Source: CAD feature listing. Evaluate the final solid. Frame: model axes, mm. A direction names the side the tool comes from. Coordinates: 2 decimals unless noted, no trailing zeros. Order: outer loops, then holes, each group sorted by start corner. A loop starts at its lowest first (then second) coordinate and runs counter-clockwise, first axis right, second up.
```python
from build123d import *

# Parameters (mm, degrees)
SKETCH1_W          = 9.5
SKETCH1_H          = 2
SKETCH1_W_2        = 9
SKETCH1_H_2        = 7
SKETCH2_W          = 4
SKETCH2_H          = 0.5
CUT_EXTRUDE1_DEPTH = 8
SKETCH3_R          = 1.25
CUT_EXTRUDE2_DEPTH = 8


with BuildPart() as part:
    # Sketch1 → Revolve1 (revolve)
    with BuildSketch(Plane.XY, mode=Mode.PRIVATE) as revolve1_sk:
        with Locations((-4.75, 1)):
            Rectangle(SKETCH1_W, SKETCH1_H)
        Polygon((0, 2), (0, 0), (21.5, 0), (21.5, 12.2), (21.5, 12.5), (2.5, 12.5), (2.5, 3.5), (0, 3.5), align=None)
        Polygon((21.5, 12.2), (21.5, 0), (52.5, 0), (52.5, 7), (52.5, 12.2), align=None)
        with Locations((57, 3.5)):
            Rectangle(SKETCH1_W_2, SKETCH1_H_2)
    revolve(revolve1_sk.sketch.rotate(Axis((0, 0, 0), (1, 0, 0)), 90), axis=Axis((0, 0, 0), (1, 0, 0)))

    # Sketch2 → Cut-Extrude1 (cut)
    with BuildSketch(Plane.ZY.offset(9.5)):
        with Locations((0, 1.75)):
            Rectangle(SKETCH2_W, SKETCH2_H)
    extrude(amount=-CUT_EXTRUDE1_DEPTH, mode=Mode.SUBTRACT)

    # Sketch3 → Cut-Extrude2 (cut)
    with BuildSketch(Plane.ZY.offset(-2.5)):
        with Locations((0, 8.5)):
            Circle(SKETCH3_R)
        with Locations(Location((0, -8.5, 0), (0, 0, 180))):
            Circle(SKETCH3_R)
    extrude(amount=-CUT_EXTRUDE2_DEPTH, mode=Mode.SUBTRACT)


solid = part.part
```
1. Section query D-D on z = -10. Return loops of the section in (x, y).
Findings:
outline: (2.5, -7.5) - (21.5, -7.5) - (21.5, -6.99) - (52.5, -6.99) - (52.5, 6.99) - (21.5, 6.99) - (21.5, 7.5) - (2.5, 7.5) - close
2. Access query for faces 1 (the face through (-9.5, 0, 0)), 2 (the face through (57.06, 6.21, 3.23)), 3 (the face through (10.5, 9, 0)). Directions: +Z, -Z, +X, -X, +Y, -Y. A direction counts if a zero-diameter tool reaches every point of the face in a straight line with its end or side. Return the directions, or none.
Findings:
face 1: +Z, -Z, -X, +Y, -Y
face 2: +X
face 3: -X
3. Draft query along Z for faces 4 (the face through (6.444, 9.554, 0.672)), 5 (the face through (-6, 1.5, 0)), 6 (the face through (36.8, 7.4, -9.7)). Return one class per face: released by +Z, released by -Z, zero draft, split by the parting line, or undercut.
Findings:
face 4: undercut
face 5: zero draft
face 6: split by the parting line
4. Section query C-C on x = 14. Return loops of the section in (y, z).
Findings:
outline: circle Ø25 at (0, 0)
5. Ray query, line 1 (Y direction, x = 6, z = 0); line 2 (X direction, y = 9, z = 2.5); line 3 (X direction, y = -3, z = -0.5). Return the intervals inside material, ascending.
Findings:
line 1: y = -12.5 to -9.75, -7.25 to 7.25, 9.75 to 12.5
line 2: x = 2.5 to 52.5
line 3: x = 0 to 61.5
6. Pin query (flat end, axial travel): P1, Ø1.5, axis at x = 13, y = -4, coming from the +Z side; P2, Ø3, axis at y = 8.5, z = 0, coming from the -X side; P3, Ø10, axis at x = 41.5, z = 7, coming from the -Y side; P4, Ø12, axis at x = 2, y = -2.5, coming from the +Z side. Return the tip coordinate at first contact, or that it passes through.
Findings:
P1: stops at z = 12.07
P2: stops at x = 2.5
P3: stops at y = -12.03
P4: stops at z = 12.5
7. Section query B-B on y = 8.5. Return loops of the section in (x, z).
Findings:
outline: (2.5, -9.17) - (21.5, -9.17) - (21.5, -8.75) - (52.5, -8.75) - (52.5, 8.75) - (21.5, 8.75) - (21.5, 9.17) - (2.5, 9.17) - (2.5, 1.25) - (10.5, 1.25) - (10.5, -1.25) - (2.5, -1.25) - close
